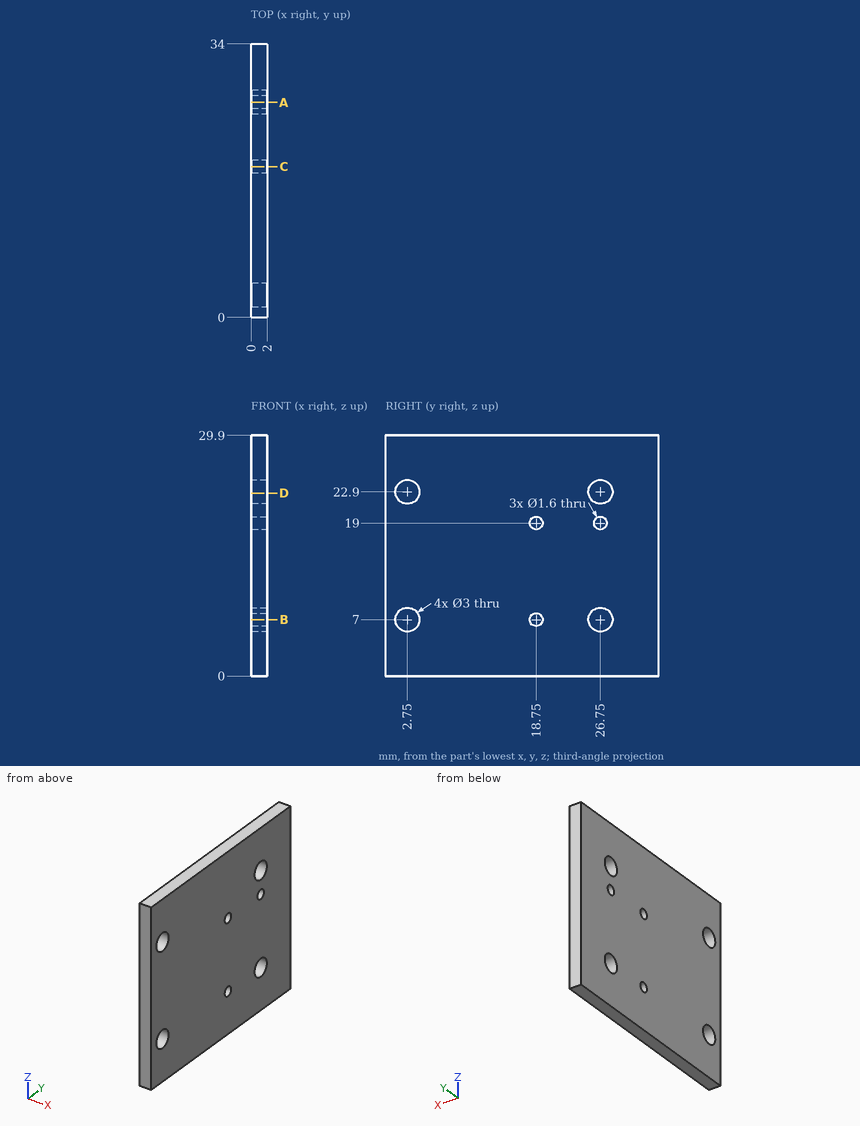
Verification items for this drawing (mm, ordinates from the low corner). Coordinates: 2 decimals unless noted, no trailing zeros. Order: outer loops, then holes, each group sorted by start corner. A loop starts at its lowest first (then second) coordinate and runs counter-clockwise, first axis right, second up. Notation, with made-up numbers: (18, 57) - (60, 57) arc R11 ccw to (60, 63) - close; hole circle Ø9 at (-33, -6.75). An arc over 180 degrees is marked (long way). Answer as a JSON object with one key per item and string values. Group by question number.
Item 1: Scan lines: probe 1 along Y at (x, z) = (1.3, 22.9); probe 2 along Y at (x, z) = (1.55, 19); probe 3 along Z at (x, y) = (0.9, 3). Record each from-to range of solid material in increasing order.
Item 2: Sectioned sample at A-A, the plane y = 26.75. Record the cut outline in (x, z), and give its area (3 significant figures).
Item 3: Sectioned sample at C-C, the plane y = 18.75. Record the cut outline in (x, z), and give its area (3 significant figures).
Item 4: Sectioned sample at D-D, the plane z = 22.75. Record the cut outline in (x, y), and give its area (3 significant figures).
Item 5: Sectioned sample at B-B, the plane z = 7. Record the cut outline in (x, y).
Resolved:
{
 "1": {"probe 1": "0 to 1.25, 4.25 to 25.25, 28.25 to 34", "probe 2": "0 to 17.95, 19.55 to 25.95, 27.55 to 34", "probe 3": "0 to 5.52, 8.48 to 21.42, 24.38 to 29.9"},
 "2": {"outline": "(0, 0) - (2, 0) - (2, 5.5) - (0, 5.5) - close; (0, 8.5) - (2, 8.5) - (2, 18.2) - (0, 18.2) - close; (0, 19.8) - (2, 19.8) - (2, 21.4) - (0, 21.4) - close; (0, 24.4) - (2, 24.4) - (2, 29.9) - (0, 29.9) - close", "area": "44.6 mm^2"},
 "3": {"outline": "(0, 0) - (2, 0) - (2, 6.2) - (0, 6.2) - close; (0, 7.8) - (2, 7.8) - (2, 18.2) - (0, 18.2) - close; (0, 19.8) - (2, 19.8) - (2, 29.9) - (0, 29.9) - close", "area": "53.4 mm^2"},
 "4": {"outline": "(0, 0) - (2, 0) - (2, 1.26) - (0, 1.26) - close; (0, 4.24) - (2, 4.24) - (2, 25.26) - (0, 25.26) - close; (0, 28.24) - (2, 28.24) - (2, 34) - (0, 34) - close", "area": "56.1 mm^2"},
 "5": {"outline": "(0, 0) - (2, 0) - (2, 1.25) - (0, 1.25) - close; (0, 4.25) - (2, 4.25) - (2, 17.95) - (0, 17.95) - close; (0, 19.55) - (2, 19.55) - (2, 25.25) - (0, 25.25) - close; (0, 28.25) - (2, 28.25) - (2, 34) - (0, 34) - close"}
}
